from build123d import *

# Parameters (mm, degrees)
SKETCH1_W           = 35.56
SKETCH1_H           = 35.56
BOSS_EXTRUDE1_DEPTH = 34
SKETCH2_R           = 5
BOSS_EXTRUDE2_DEPTH = 24
SKETCH3_R           = 5
BOSS_EXTRUDE3_DEPTH = 12
SKETCH4_R           = 2
CUT_EXTRUDE1_DEPTH  = 34


with BuildPart() as part:
    # Sketch1 → Boss-Extrude1 (new body)
    with BuildSketch(Plane(origin=(0, 0, 0), x_dir=(1, 0, 0), z_dir=(0, 1, 0))):
        Rectangle(SKETCH1_W, SKETCH1_H)
    extrude(amount=BOSS_EXTRUDE1_DEPTH)

    # Sketch2 → Boss-Extrude2 (add)
    with BuildSketch(Plane(origin=(0, 34, 0), x_dir=(1, 0, 0), z_dir=(0, 1, 0))):
        Circle(SKETCH2_R)
    extrude(amount=BOSS_EXTRUDE2_DEPTH)

    # Sketch3 → Boss-Extrude3 (add)
    with BuildSketch(Plane.XZ):
        Circle(SKETCH3_R)
    extrude(amount=BOSS_EXTRUDE3_DEPTH)

    # Sketch4 → Cut-Extrude1 (cut)
    with BuildSketch(Plane(origin=(0, 34, 0), x_dir=(1, 0, 0), z_dir=(0, 1, 0))):
        with Locations((-13, 13)):
            Circle(SKETCH4_R)
        with Locations((13, 13)):
            Circle(SKETCH4_R)
        with Locations((13, -13)):
            Circle(SKETCH4_R)
        with Locations((-13, -13)):
            Circle(SKETCH4_R)
    extrude(amount=-CUT_EXTRUDE1_DEPTH, mode=Mode.SUBTRACT)


solid = part.part
Check sheet for the modelled part. Datum: model origin and axes. Units: mm. A direction names the side the tool comes from. Round coordinates to 2 decimals unless told otherwise and drop trailing zeros. Order: outer loops, then holes, each group sorted by start corner. A loop starts at its lowest first (then second) coordinate and runs counter-clockwise, first axis right, second up.
(1) Cross-section at B-B, the plane x = 13. Enter the section's corners in (y, z).
(2) Cross-section at C-C, the plane y = 19.5. Enter the section's corners in (x, z), and give its area (3 significant figures).
(3) Cross-section at D-D, the plane x = 0. Enter the section's corners in (y, z).
(4) Cross-section at A-A, the plane z = -13. Enter the section's corners in (x, y).
(5) Access from +Z, -Z, +X, -X, +Y, -Y to the whole of each face (thin tool, end or side, straight path). Record for faces 1 (the flat face through (4, 34, -4)), 2 (the cylindrical face through (-1.08, -5.92, -4.88)), 3 (the flat face through (0, 58, 0)).
(6) Go/stop test with flat-tipped pins: P1, Ø10.5, axis at x = -6, z = 2.5, coming from the -Y side; P2, Ø12, axis at y = 47, z = -5.5, coming from the +X side; P3, Ø6.5, axis at x = -13, z = 13, coming from the +Y side; P4, Ø5, axis at x = -11.5, z = 3.5, coming from the -Y side. Record where each tip stops, or that it passes through.
(7) Scan lines: probe 1 along Z at (x, y) = (-13, 18); probe 2 along Z at (x, y) = (-11.5, 18.5). Record each from-to range of solid material in increasing order.
(8) Draft check along X on faces 4 (the flat face through (0, 17, -17.78)), 5 (the cylindrical face through (-14.474, 17.238, -14.352)), 6 (the flat face through (17.78, 17, 0)). Enter one of: pulls with the +X half, pulls with the -X half, needs draft (parallel to the pull), parting line crosses it, or undercut.
Check sheet entries:
1. outline: (0, -17.78) - (34, -17.78) - (34, -15) - (0, -15) - close; (0, -11) - (34, -11) - (34, 11) - (0, 11) - close; (0, 15) - (34, 15) - (34, 17.78) - (0, 17.78) - close
2. outline: (-17.78, -17.78) - (17.78, -17.78) - (17.78, 17.78) - (-17.78, 17.78) - close; hole circle Ø4 at (-13, -13); hole circle Ø4 at (-13, 13); hole circle Ø4 at (13, -13); hole circle Ø4 at (13, 13)
2. area: 1,210 mm2
3. outline: (-12, -5) - (0, -5) - (0, -17.78) - (34, -17.78) - (34, -5) - (58, -5) - (58, 5) - (34, 5) - (34, 17.78) - (0, 17.78) - (0, 5) - (-12, 5) - close
4. outline: (-17.78, 0) - (-15, 0) - (-15, 34) - (-17.78, 34) - close; (-11, 0) - (11, 0) - (11, 34) - (-11, 34) - close; (15, 0) - (17.78, 0) - (17.78, 34) - (15, 34) - close
5. face 1: +Y
5. face 2: -Y
5. face 3: +Z, -Z, +X, -X, +Y
6. P1: stops at y = -12
6. P2: stops at x = 5
6. P3: stops at y = 34
6. P4: stops at y = 0
7. probe 1: z = -17.78 to -15, -11 to 11, 15 to 17.78
7. probe 2: z = -17.78 to -14.32, -11.68 to 11.68, 14.32 to 17.78
8. face 4: needs draft
8. face 5: undercut
8. face 6: pulls with the +X half
